Read the model definition and answer for the solid it produces. Units are mm, in the model's axes. A direction names the side the tool comes from. Give positions to 0.01 mm unless a question says otherwise; leave off trailing zeros. Write each loop counter-clockwise with the first axis right and the second up, starting at its lowest first coordinate (ties: lowest second). Pieces come first, ordered by that corner, then holes. Notation, with made-up numbers: (84.5, 16.5) -> (88.5, 16.5) arc R10 cw to (88.5, 30.5) -> close; hole circle Ø4 at (29, 47). An arc over 180 degrees is marked (long way). Put each result on its own line as item: value. Start each with the question number.
from build123d import *

# Parameters (mm, degrees)
SKETCH005_W     = 122.986
SKETCH005_H     = 21.18
SKETCH005_W_2   = 119.986
SKETCH005_H_2   = 18.18
PAD004_DEPTH    = 9.9
SKETCH006_W     = 122.986
SKETCH006_H     = 21.18
PAD005_DEPTH    = 1.5
SKETCH007_W     = 13.9
SKETCH007_H     = 14.3
POCKET001_DEPTH = 9.901
SKETCH008_R     = 1.45
SKETCH008_W     = 1.5
SKETCH008_H     = 18.18
PAD006_DEPTH    = 3.5
SKETCH009_W     = 9
SKETCH009_H     = 2
SKETCH009_W_2   = 17
PAD007_DEPTH    = 2
POCKET002_DEPTH = 6.5
FILLET_R        = 1
PAD008_DEPTH    = 18.18
SKETCH012_W     = 50
SKETCH012_H     = 5
POCKET003_DEPTH = 1
CHAMFER001_SIZE = 0.5
SKETCH013_R     = 1.45
POCKET004_DEPTH = 1


with BuildPart() as part:
    # Sketch005 (on ShapeBinder) → Pad004 (new body)
    with BuildSketch(Plane(origin=(-93.484762, 101.426, -4.5), x_dir=(1, 0, 0), z_dir=(0, 0, -1))):
        with Locations((153.277762, 92.79)):
            Rectangle(SKETCH005_W, SKETCH005_H)
        with Locations((153.277762, 92.79)):
            Rectangle(SKETCH005_W_2, SKETCH005_H_2, mode=Mode.SUBTRACT)
    extrude(amount=-PAD004_DEPTH)

    # Sketch006 (on Face10 of Pad004) → Pad005 (join)
    with BuildSketch(Plane(origin=(-93.484762, 101.426, 5.4), x_dir=(1, 0, 0), z_dir=(0, 0, 1))):
        with Locations((153.277762, -92.79)):
            Rectangle(SKETCH006_W, SKETCH006_H)
    extrude(amount=-PAD005_DEPTH)

    # Sketch007 (on Face16 of Pad005) → Pocket001 (cut, through all)
    with BuildSketch(Plane(origin=(-93.484762, 101.426, 5.4), x_dir=(1, 0, 0), z_dir=(0, 0, 1))):
        with Locations((101.358762, -92.79)):
            Rectangle(SKETCH007_W, SKETCH007_H)
        with Locations((125.158762, -92.79)):
            Rectangle(SKETCH007_W, SKETCH007_H)
        with Locations((148.958762, -92.79)):
            Rectangle(SKETCH007_W, SKETCH007_H)
        with Locations((172.758762, -92.79)):
            Rectangle(SKETCH007_W, SKETCH007_H)
    extrude(amount=-POCKET001_DEPTH, mode=Mode.SUBTRACT)

    # Sketch008 (on Face15 of Pocket001) → Pad006 (join)
    with BuildSketch(Plane(origin=(-93.484762, 101.426, 3.9), x_dir=(1, 0, 0), z_dir=(0, 0, -1))):
        with BuildLine():
            Line((112.483762, 96.208699), (112.483762, 101.88))
            Line((112.483762, 101.88), (113.983762, 101.88))
            Line((113.983762, 101.88), (113.983762, 96.208699))
            ThreePointArc((113.983762, 89.371301), (116.733762, 92.79), (113.983762, 96.208699))
            Line((113.983762, 83.7), (113.983762, 89.371301))
            Line((112.483762, 83.7), (113.983762, 83.7))
            Line((112.483762, 83.7), (112.483762, 89.371301))
            ThreePointArc((112.483762, 96.208699), (109.733762, 92.79), (112.483762, 89.371301))
        make_face()
        with Locations((113.233762, 92.79)):
            Circle(SKETCH008_R, mode=Mode.SUBTRACT)
        with Locations((136.983762, 92.79)):
            Rectangle(SKETCH008_W, SKETCH008_H)
        with BuildLine():
            Line((159.983762, 101.88), (161.483762, 101.88))
            Line((161.483762, 101.88), (161.483762, 96.208699))
            ThreePointArc((161.483762, 89.371301), (164.233762, 92.79), (161.483762, 96.208699))
            Line((161.483762, 83.7), (161.483762, 89.371301))
            Line((159.983762, 83.7), (161.483762, 83.7))
            Line((159.983762, 83.7), (159.983762, 89.371301))
            ThreePointArc((159.983762, 96.208699), (157.233762, 92.79), (159.983762, 89.371301))
            Line((159.983762, 101.88), (159.983762, 96.208699))
        make_face()
        with Locations((160.733762, 92.79)):
            Circle(SKETCH008_R, mode=Mode.SUBTRACT)
    extrude(amount=PAD006_DEPTH)

    # Sketch009 (on Face27 of Pad006) → Pad007 (join)
    with BuildSketch(Plane(origin=(-93.484762, 101.426, 3.9), x_dir=(1, 0, 0), z_dir=(0, 0, -1))):
        with Locations((195.770762, 84.7)):
            Rectangle(SKETCH009_W, SKETCH009_H)
        with Locations((191.770762, 100.88)):
            Rectangle(SKETCH009_W_2, SKETCH009_H)
    extrude(amount=PAD007_DEPTH)

    # Sketch010 (on Face5 of Pad007) → Pocket002 (cut)
    with BuildSketch(Plane(origin=(121.286, 101.426, -1.6), x_dir=(0, 1, 0), z_dir=(1, 0, 0))):
        with BuildLine():
            ThreePointArc((-95.29, 6.5), (-97.04, 4.75), (-95.29, 3))
            Line((-95.29, 3), (-90.29, 3))
            ThreePointArc((-90.29, 3), (-88.54, 4.75), (-90.29, 6.5))
            Line((-95.29, 6.5), (-90.29, 6.5))
        make_face()
    extrude(amount=-POCKET002_DEPTH, mode=Mode.SUBTRACT)

    # Fillet
    fillet_edges = [part.edges().sort_by_distance(p)[0] for p in [
        (121.286, 19.226, -0.3),
        (121.286, -1.954, -0.3),
        (-1.7, 19.226, -0.3),
        (-1.7, -1.954, -0.3),
    ]]
    fillet(fillet_edges, radius=FILLET_R)

    # Sketch011 (on Face14 of Fillet) → Pad008 (join)
    with BuildSketch(Plane(origin=(-93.484762, -0.454, -1.6), x_dir=(-1, 0, 0), z_dir=(0, 1, 0))):
        with BuildLine():
            ThreePointArc((-213.270762, -1.1), (-212.070762, 0.1), (-213.270762, 1.3))
            Line((-213.270762, 1.3), (-213.270762, -1.1))
        make_face()
    extrude(amount=PAD008_DEPTH)

    # Sketch012 (on Face1 of Pad008) → Pocket003 (cut)
    with BuildSketch(Plane(origin=(-93.484762, 19.226, -1.6), x_dir=(-1, 0, 0), z_dir=(0, 1, 0))):
        with Locations((-137.058762, 2.05)):
            Rectangle(SKETCH012_W, SKETCH012_H)
    extrude(amount=-POCKET003_DEPTH, mode=Mode.SUBTRACT)

    # Chamfer001
    chamfer001_edges = [part.edges().sort_by_distance(p)[0] for p in [
        (43.574, 19.226, -2.05),
        (68.574, 19.226, 0.45),
        (43.574, 19.226, 2.95),
        (18.574, 19.226, 0.45),
    ]]
    chamfer(chamfer001_edges, length=CHAMFER001_SIZE)

    # Sketch013 (on Face87 of Chamfer001) → Pocket004 (cut)
    with BuildSketch(Plane(origin=(-93.484762, 101.426, 3.9), x_dir=(1, 0, 0), z_dir=(0, 0, -1))):
        with Locations((113.233762, 92.79)):
            Circle(SKETCH013_R)
        with Locations((160.733762, 92.79)):
            Circle(SKETCH013_R)
    extrude(amount=-POCKET004_DEPTH, mode=Mode.SUBTRACT)


solid = part.part
1) For faces 5 (the face through (48, 9, 3.9)), 6 (the face through (121.286, 9, -1)), 7 (the face through (44, 18.226, 0)), determine the directions among +Z, -Z, +X, -X, +Y, -Y from which every point of the face is accessible in a straight line to the end or side of a thin tool.
2) Each of these flat-tipped pins is pushed along its axis until it touches: pin 1 Ø1.6 at (y, z) = (11, 4.5) entering from +X; pin 2 Ø2 at (x, y) = (103.5, 16.5) entering from -Z; pin 3 Ø1.2 at (x, y) = (43, 8) entering from -Z. Where does it stop, or does it pass through?
3) A cutting plane is placed at D-D on x = 77.5. Give the vertices of the cut face in (y, z).
4) For a pull along Y with two mould halves and no side action, classify faces 1 (the face through (70.75, 8.7, 2.17)), 2 (the face through (60, -1, -4.5)), 3 (the face through (-0.2, 9, 0)), 4 (the face through (72, 19.226, 0)) as pulls with the +Y half, pulls with the -Y half, needs draft (parallel to the pull), parting line crosses it, or undercut.
5) Straight lines are drawn through the part: line 1 (X direction, y = 1, z = 1.5); line 2 (X direction, y = 2.75, z = -2.75); line 3 (Y direction, x = 65, z = -3.25). For each, find the intervals that lie inside material, in ascending order. Write a range as [from, to].
6) A cutting plane is placed at C-C on y = 2.75. State how many separate pieces and enclosed holes the cut face has, and give its area (3 significant figures).
7) A cutting plane is placed at B-B on x = 91. Give the vertices of the cut face in (y, z), and give its area (3 significant figures).
8) A cutting plane is placed at A-A on x = 30.5. Give the vertices of the cut face in (y, z), and give its area (3 significant figures).
Results found:
1. face 5: -Z
1. face 6: +Z, -Z, +X, +Y, -Y
1. face 7: +Y
2. pin 1: stops at x = 121.29
2. pin 2: stops at z = 1.9
2. pin 3: stops at z = 0.4
3. outline: (-1.95, -4.5) -> (-0.45, -4.5) -> (-0.45, 3.9) -> (1.49, 3.9) -> (1.49, 5.4) -> (-1.95, 5.4) -> close; (15.79, 3.9) -> (17.73, 3.9) -> (17.73, -4.5) -> (19.23, -4.5) -> (19.23, 5.4) -> (15.79, 5.4) -> close
4. face 1: undercut
4. face 2: needs draft
4. face 3: undercut
4. face 4: pulls with the +Y half
5. line 1: x = [-1.7, -0.2], [19, 20.5], [42.75, 44.25], [66.5, 68], [119.79, 121.29]
5. line 2: x = [-1.7, -0.2], [119.79, 121.29]
5. line 3: y = [-1.95, -0.45], [17.73, 19.23]
6. separate pieces: 5
6. enclosed holes: 0
6. area: 144 mm²
7. outline: (-1.95, -4.5) -> (-0.45, -4.5) -> (-0.45, 1.9) -> (1.55, 1.9) -> (1.55, 3.9) -> (17.73, 3.9) -> (17.73, -4.5) -> (19.23, -4.5) -> (19.23, 5.4) -> (-1.95, 5.4) -> close
7. area: 61.0 mm²
8. outline: (-1.95, -4.5) -> (-0.45, -4.5) -> (-0.45, 3.9) -> (1.49, 3.9) -> (1.49, 5.4) -> (-1.95, 5.4) -> close; (15.79, 3.9) -> (17.73, 3.9) -> (17.73, -4.5) -> (19.23, -4.5) -> (19.23, -2.55) -> (18.73, -2.05) -> (18.23, -2.05) -> (18.23, 2.95) -> (18.73, 2.95) -> (19.23, 3.45) -> (19.23, 5.4) -> (15.79, 5.4) -> close
8. area: 30.3 mm²
